The drawing under review shows one solid part. Ordinate dimensions are in mm from its lowest x, y, z. A direction names the side the tool comes from. Coordinates: 2 decimals unless noted, no trailing zeros. Loops run counter-clockwise (first coordinate to the right, second up) from the corner with the lowest first, then second, coordinate; pieces in that order, holes last. Notation, with made-up numbers: (25, -37.5) - (39, -37.5) arc R27 ccw to (39, -18.5) - close; hole circle Ø8 at (-17.5, 38.25). An arc over 180 degrees is marked (long way). Answer as a JSON object with one key per item and string values. Group by question number.
Item 1: To check wall thickness, follow line 1 (Z direction, x = 34, y = 62.5); line 2 (X direction, y = 33.5, z = 68); line 3 (X direction, y = 10.5, z = 28.5) (1 decimal). State the ranges of each line that lie inside material, in increasing order.
Item 2: We need section C-C (x = 52). Give the boundary of the cut face in (y, z), then the cut area to 3 significant figures.
Item 3: Clearance check with flat-ended pins moving along their axes: pin 1 (6 mm diameter, centred on x = 17, y = 43, fed in from -Z); pin 2 (8 mm diameter, centred on x = 36, z = 41, fed in from -Y); pin 3 (8 mm diameter, centred on x = 50.5, z = 10.5, fed in from -Y) (1 decimal). State where each tip first meets the part, or that it passes through.
Item 4: Tool access review of the marked faces 1, 2 and 3: name each direction out of +Z, -Z, +X, -X, +Y, -Y from which nothing blocks a thin tool from reaching the whole face with its end or side.
Item 5: We need section B-B (z = 6.5). Give the boundary of the cut face in (x, y).
Item 6: We need section A-A (y = 57.5). Give the boundary of the cut face in (x, z), then the cut area to 3 significant figures.
Item 7: We need section D-D (z = 34.5). Give the boundary of the cut face in (x, y) (1 decimal), then the cut area to 3 significant figures.
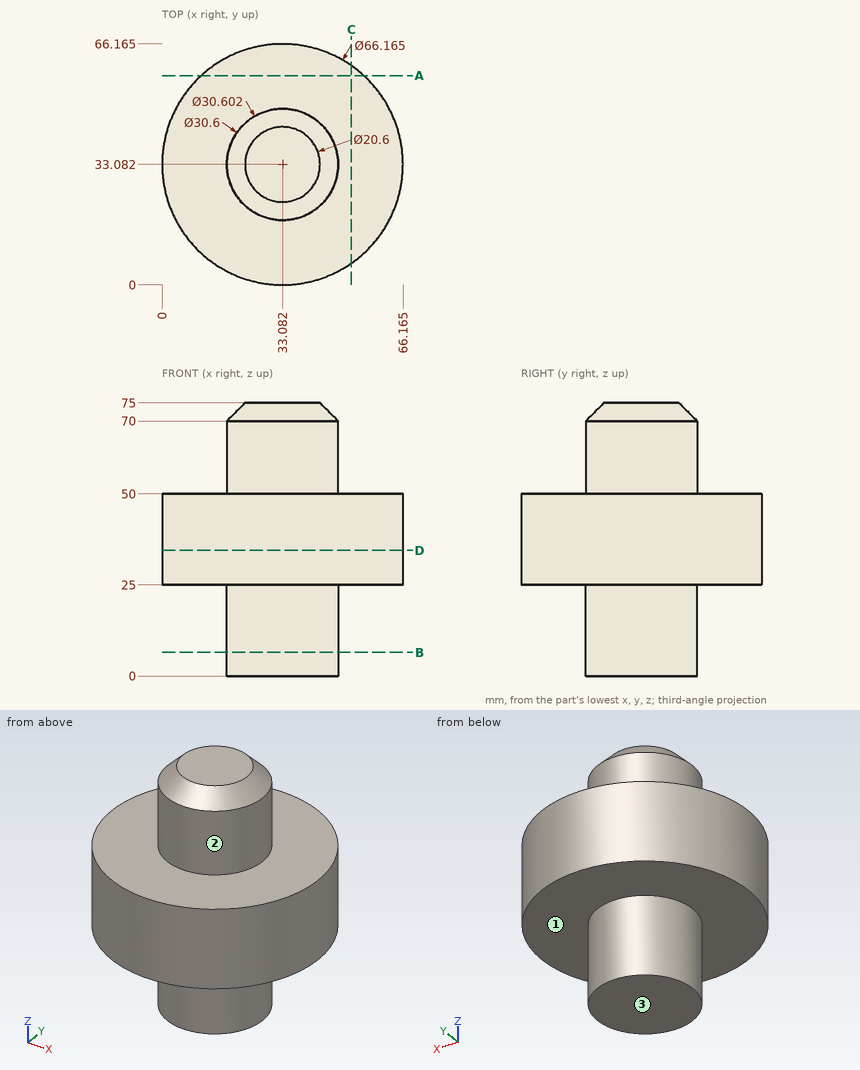
Check sheet entries:
{
 "1": {"line 1": "z = 25 to 50", "line 2": "x = 17.79 to 48.38", "line 3": "x = 8.9 to 57.3"},
 "2": {"outline": "(5.94, 25) - (60.22, 25) - (60.22, 50) - (5.94, 50) - close", "area": "1,360 mm2"},
 "3": {"pin 1": "stops at z = 25", "pin 2": "stops at y = 0", "pin 3": "stops at y = 25.7"},
 "4": {"face 1": "-Z", "face 2": "+Z", "face 3": "-Z, +X, -X, +Y, -Y"},
 "5": {"outline": "circle Ø30.6 at (33.08, 33.08)"},
 "6": {"outline": "(10.76, 25) - (55.4, 25) - (55.4, 50) - (10.76, 50) - close", "area": "1,120 mm2"},
 "7": {"outline": "circle Ø66.2 at (33.1, 33.1)", "area": "3,440 mm2"}
}
